The listing builds one solid part. Answer for the finished solid, in the listing's coordinates (mm). Face numbers are marked on the shaded views. A direction names the side the tool comes from. Coordinates: 2 decimals unless noted, no trailing zeros. Loops run counter-clockwise (first coordinate to the right, second up) from the corner with the lowest first, then second, coordinate; pieces in that order, holes last. Notation, with made-up numbers: M 42.5,65 L 67.5,65 A26 ccw 67.5,98 Z; hole C -25.5,-1 d4. An arc over 180 degrees is marked long. Answer as a JSON object with one key per item and string values. Group by question number.
1. A cutting plane is placed at D-D on z = 6.5. Give the vertices of the cut face in (x, y) (3 decimals).
2. Given pin 1 (4 mm diameter, centred on x = 10, y = 5, fed in from +Z); pin 2 (3.5 mm diameter, centred on x = 16, z = 7.5, fed in from +Y), each flat-ended and moving along its own axis, determine where each tip first touches the part or whether it passes through.
3. For the marked faces 1 and 2, determine the directions among +Z, -Z, +X, -X, +Y, -Y from which every point of the face is accessible in a straight line to the end or side of a thin tool.
4. A cutting plane is placed at C-C on z = 2.5. Give the vertices of the cut face in (x, y).
5. Straight lines are drawn through the part: L1, parallel to X at y = 8.75, z = 3.75; L2, parallel to X at y = 9.75, z = 6; L3, parallel to Y at x = 30, z = 0.6. For each, find the intervals that lie inside material, in ascending order.
6. A cutting plane is placed at A-A on x = 31. Give the vertices of the cut face in (y, z).
7. A cutting plane is placed at B-B on y = 7. Give the vertices of the cut face in (x, z).
8. Determine the mould class of the marked faces 3, 4, 5 and 6 for opening direction X: released by +X, released by -X, zero draft, split by the parting line, or undercut.
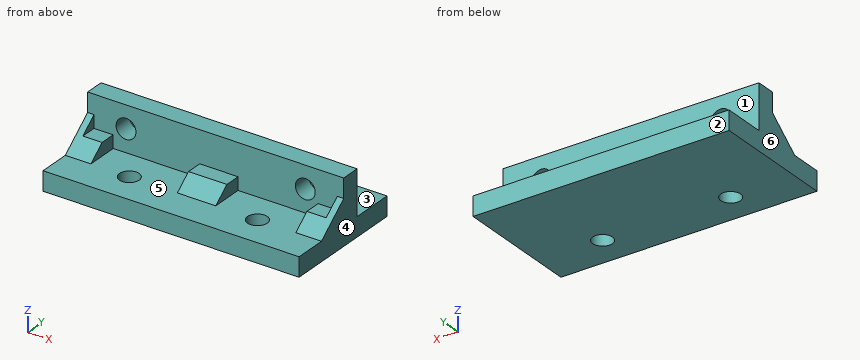
from build123d import *

# Parameters (mm, degrees)
SKETCH_1_W          = 40
SKETCH_1_H          = 6.7
EXTRUDE_1_DEPTH     = 3
EXTRUDE_2_DEPTH     = 3
SKETCH_1_5_W        = 40
SKETCH_1_5_H        = 3
EXTRUDE_3_DEPTH     = 10
CUT_EXTRUDE_1_DEPTH = 3
SKETCH_3_W          = 3
SKETCH_3_H          = 2
SKETCH_3_W_2        = 1
EXTRUDE_4_DEPTH     = 5
CUT_EXTRUDE_2_DEPTH = 44


with BuildPart() as part:
    # Sketch 1 → Extrude 1 (new body)
    with BuildSketch(Plane.XY):
        with Locations((20, 16.35)):
            Rectangle(SKETCH_1_W, SKETCH_1_H)
    extrude(amount=EXTRUDE_1_DEPTH)



with BuildPart() as body_2:
    # Sketch 1_3 → Extrude 2 (new body)
    with BuildSketch(Plane.XY):
        with BuildLine():
            Line((20, 5), (11.55, 5))
            ThreePointArc((11.55, 5), (10, 3.45), (8.45, 5))
            Line((8.45, 5), (0, 5))
            Line((0, 5), (0, 0))
            Line((0, 0), (40, 0))
            Line((40, 0), (40, 5))
            Line((40, 5), (31.55, 5))
            ThreePointArc((31.55, 5), (30, 3.45), (28.45, 5))
            Line((28.45, 5), (20, 5))
        make_face()
        with BuildLine():
            ThreePointArc((8.45, 5), (10, 6.55), (11.55, 5))
            Line((11.55, 5), (20, 5))
            Line((20, 5), (28.45, 5))
            ThreePointArc((28.45, 5), (30, 6.55), (31.55, 5))
            Line((31.55, 5), (40, 5))
            Line((40, 5), (40, 10))
            Line((40, 10), (0, 10))
            Line((0, 10), (0, 5))
            Line((0, 5), (8.45, 5))
        make_face()
    extrude(amount=EXTRUDE_2_DEPTH)


with BuildPart() as part_1:
    add(part.part)

    add(body_2.part)  # Extrude 3 merges body 2
    # Sketch 1_5 → Extrude 3 (add)
    with BuildSketch(Plane.XY):
        with Locations((20, 11.5)):
            Rectangle(SKETCH_1_5_W, SKETCH_1_5_H)
    extrude(amount=EXTRUDE_3_DEPTH)

    # Sketch 2 → Cut-Extrude 1 (cut)
    with BuildSketch(Plane(origin=(0, 13, 0), x_dir=(1, 0, 0), z_dir=(0, 1, 0))):
        with BuildLine():
            Line((4.45, -6.5), (6, -6.5))
            Line((6, -6.5), (7.55, -6.5))
            ThreePointArc((7.55, -6.5), (6, -4.95), (4.45, -6.5))
        make_face()
        with BuildLine():
            Line((7.55, -6.5), (6, -6.5))
            Line((6, -6.5), (4.45, -6.5))
            ThreePointArc((4.45, -6.5), (6, -8.05), (7.55, -6.5))
        make_face()
        with BuildLine():
            ThreePointArc((35.55, -6.5), (34, -4.95), (32.45, -6.5))
            Line((32.45, -6.5), (34, -6.5))
            Line((34, -6.5), (35.55, -6.5))
        make_face()
        with BuildLine():
            Line((34, -6.5), (32.45, -6.5))
            ThreePointArc((32.45, -6.5), (34, -8.05), (35.55, -6.5))
            Line((35.55, -6.5), (34, -6.5))
        make_face()
    extrude(amount=-CUT_EXTRUDE_1_DEPTH, mode=Mode.SUBTRACT)

    # Sketch 3 → Extrude 4 (add)
    with BuildSketch(Plane.XZ.offset(-10)):
        Polygon((17.5, 5), (17.5, 3), (23.5, 3), (23.5, 5), (20.5, 5), align=None)
        Polygon((0, 5), (0, 3), (1, 3), (4, 3), (4, 5), (2, 5), (1, 5), (1, 7), (0, 7), align=None)
        with Locations((37.5, 4)):
            Rectangle(SKETCH_3_W, SKETCH_3_H)
        with Locations((39.5, 4)):
            Rectangle(SKETCH_3_W_2, SKETCH_3_H)
        with Locations((39.5, 6)):
            Rectangle(SKETCH_3_W_2, SKETCH_3_H)
    extrude(amount=EXTRUDE_4_DEPTH)

    # Sketch 4 → Cut-Extrude 2 (cut)
    with BuildSketch(Plane.ZY):
        Polygon((7, 10), (3, 5), (7, 5), align=None)
    extrude(amount=-CUT_EXTRUDE_2_DEPTH, mode=Mode.SUBTRACT)


solid = part_1.part
From the geometry:
{
 "1": {"outline": "M 0,9.375 L 1,9.375 L 1,10 L 4.45,10 L 4.45,13 L 0,13 Z; M 7.55,10 L 32.45,10 L 32.45,13 L 7.55,13 Z; M 35.55,10 L 39,10 L 39,9.375 L 40,9.375 L 40,13 L 35.55,13 Z"},
 "2": {"pin 1": "stops at z = 3", "pin 2": "stops at y = 13"},
 "3": {"face 1": "+Z, +X, -X, +Y", "face 2": "+Z, -Z, +X, -X, +Y"},
 "4": {"outline": "M 0,0 L 40,0 L 40,19.7 L 0,19.7 Z; hole C 10,5 d3.1; hole C 30,5 d3.1"},
 "5": {"L1": "x = 0 to 4, 17.5 to 23.5, 36 to 40", "L2": "x = 0 to 1, 39 to 40", "L3": "y = 0 to 3.45, 6.55 to 19.7"},
 "6": {"outline": "M 0,0 L 3.82,0 L 3.82,3 L 0,3 Z; M 6.18,0 L 19.7,0 L 19.7,3 L 13,3 L 13,10 L 10,10 L 10,3 L 6.18,3 Z"},
 "7": {"outline": "M 0,0 L 40,0 L 40,4.6 L 36,4.6 L 36,3 L 23.5,3 L 23.5,4.6 L 17.5,4.6 L 17.5,3 L 4,3 L 4,4.6 L 0,4.6 Z"},
 "8": {"face 3": "zero draft", "face 4": "released by +X", "face 5": "undercut", "face 6": "released by -X"}
}
